For this review, use the dimensioned drawing (mm, ordinates from the lowest corner) and the shaded views. A direction names the side the tool comes from. Give positions to 0.01 mm unless a question says otherwise; leave off trailing zeros. Order: outer loops, then holes, each group sorted by start corner. A loop starts at its lowest first (then second) coordinate and runs counter-clockwise, first axis right, second up.
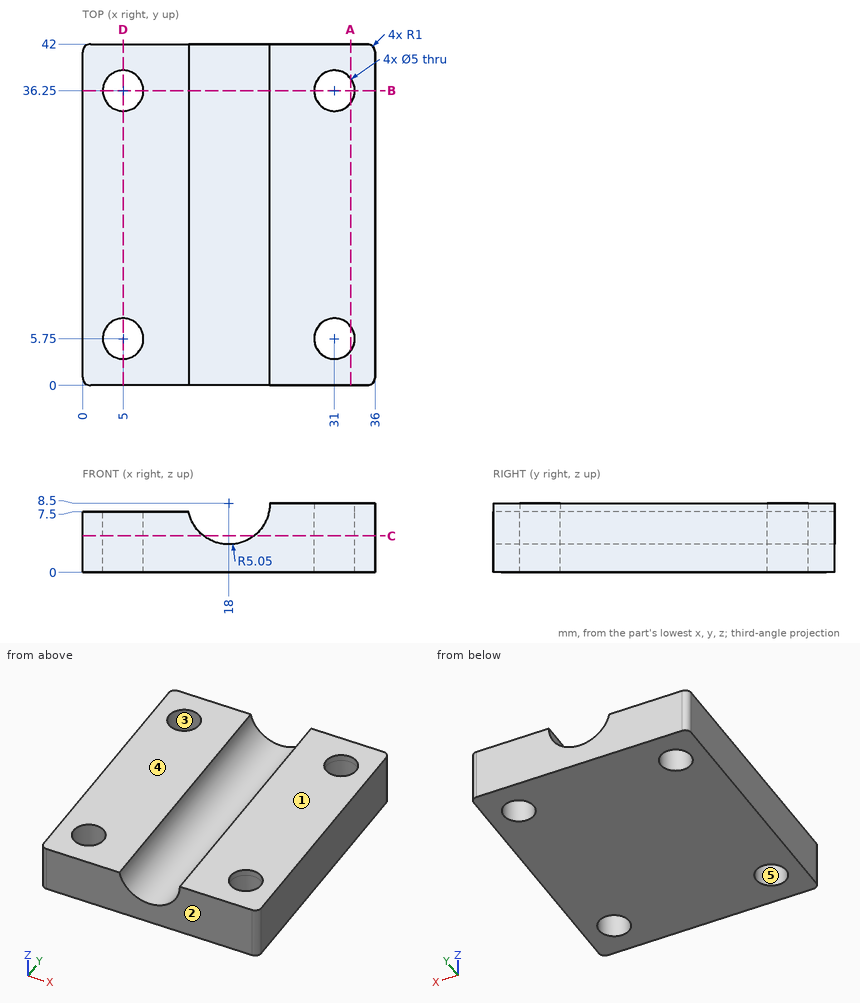
1. For pin 1 (8 mm diameter, centred on x = 31, y = 5.75, fed in from -Z); pin 2 (4 mm diameter, centred on x = 5, y = 5.75, fed in from +Z); pin 3 (14.5 mm diameter, centred on x = 5, y = 28.5, fed in from +Z), all flat-tipped, find the tip position at first contact; note any pin that passes through.
Recorded:
pin 1: stops at z = 0
pin 2: passes through
pin 3: stops at z = 7.5
2. Draft analysis for pull direction Y (two halves, no side actions). For the marked faces 1, 2 and 3, state which applies: pulls with the +Y half, pulls with the -Y half, needs draft (parallel to the pull), parting line crosses it, or undercut.
Recorded:
face 1: needs draft
face 2: pulls with the -Y half
face 3: undercut
3. Take a section at D-D (x = 5). State the section outline as (y, z) points, then the cut area to 3 significant figures.
Recorded:
outline: (0, 0) - (3.25, 0) - (3.25, 7.5) - (0, 7.5) - close; (8.25, 0) - (33.75, 0) - (33.75, 7.5) - (8.25, 7.5) - close; (38.75, 0) - (42, 0) - (42, 7.5) - (38.75, 7.5) - close
area: 240 mm2
4. Machinability: for the marked faces 4 and 5, which of the approach directions +Z, -Z, +X, -X, +Y, -Y give a long, thin tool a straight path to every point of the face, cutting with its end or side? Answer none if there is none.
Recorded:
face 4: +Z, -X, +Y, -Y
face 5: +Z, -Z
5. Take a section at B-B (y = 36.25). State the section outline as (x, z) points.
Recorded:
outline: (0, 0) - (2.5, 0) - (2.5, 7.5) - (0, 7.5) - close; (7.5, 0) - (28.5, 0) - (28.5, 8.5) - (23.05, 8.5) arc R5.05 cw to (13.05, 7.5) - (7.5, 7.5) - close; (33.5, 0) - (36, 0) - (36, 8.5) - (33.5, 8.5) - close
6. For line 1 along Y through (x, z) = (31, 8.1); line 2 along X through (y, z) = (5.75, 1.5); line 3 along Y through (x, z) = (32.5, 7.75), list the stretches that pass through material, from the lowest coordinate up.
Recorded:
line 1: y = 0 to 3.25, 8.25 to 33.75, 38.75 to 42
line 2: x = 0 to 2.5, 7.5 to 28.5, 33.5 to 36
line 3: y = 0 to 3.75, 7.75 to 34.25, 38.25 to 42
7. Take a section at A-A (x = 33). State the section outline as (y, z) points.
Recorded:
outline: (0, 0) - (4.25, 0) - (4.25, 8.5) - (0, 8.5) - close; (7.25, 0) - (34.75, 0) - (34.75, 8.5) - (7.25, 8.5) - close; (37.75, 0) - (42, 0) - (42, 8.5) - (37.75, 8.5) - close
8. Take a section at C-C (z = 4.5). State the section outline as (x, y) points, then the cut area to 3 significant figures.
Recorded:
outline: (0, 1) arc R1 ccw to (1, 0) - (14.92, 0) - (14.92, 42) - (1, 42) arc R1 ccw to (0, 41) - close; (21.08, 0) - (35, 0) arc R1 ccw to (36, 1) - (36, 41) arc R1 ccw to (35, 42) - (21.08, 42) - close; hole circle Ø5 at (5, 5.75); hole circle Ø5 at (5, 36.25); hole circle Ø5 at (31, 5.75); hole circle Ø5 at (31, 36.25)
area: 1,170 mm2
